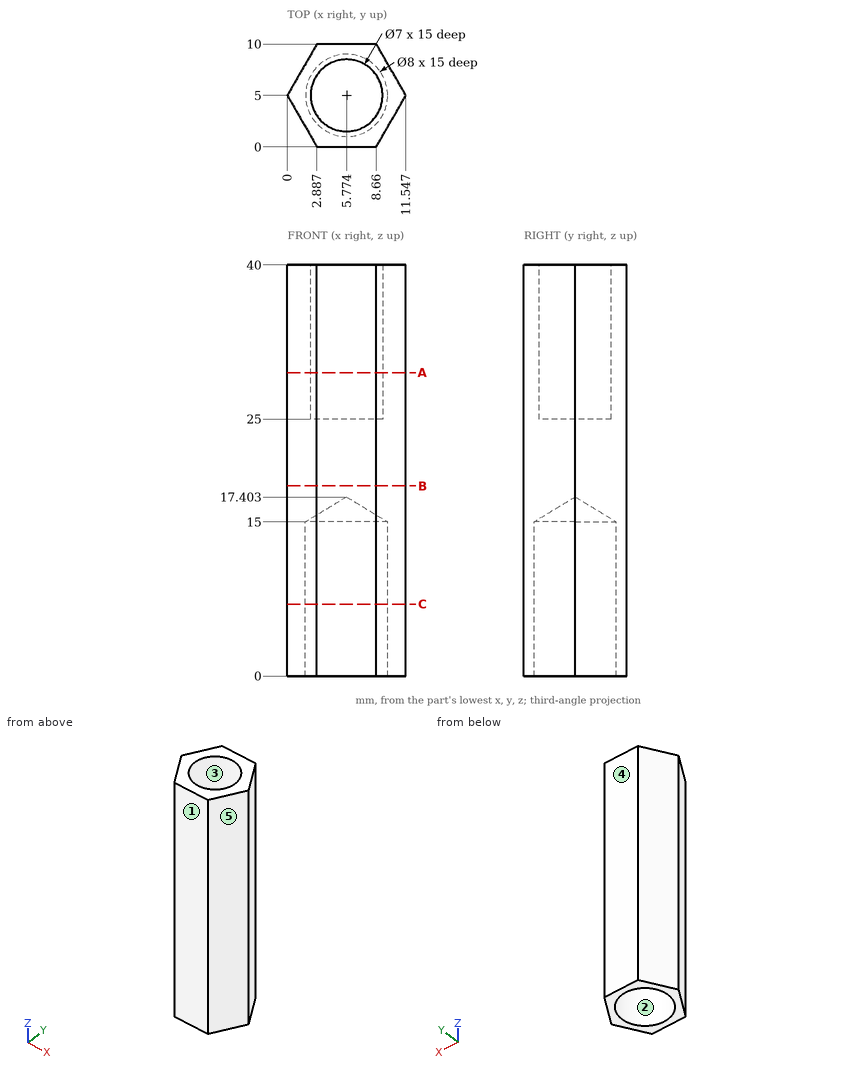
Here's the drawing with two shaded views (mm, measured from the low corner). I have some questions. A direction names the side the tool comes from. Coordinates: 2 decimals unless noted, no trailing zeros. Write each loop counter-clockwise with the first axis right and the second up, starting at its lowest first coordinate (ties: lowest second). Pieces come first, ordered by that corner, then holes. Notation, with made-up numbers: M -27,-25 L 17,-25 A29 cw 17,7 Z; hole C -9.5,4 d2. An arc over 180 degrees is marked long. Answer as CSV lines item,"result".
Item 1: Imagine slicing it at C-C on z = 7. List the corners of the cut face in (x, y) for me.
Geometry results:
outline,"M 0,5 L 2.89,0 L 8.66,0 L 11.55,5 L 8.66,10 L 2.89,10 Z; hole C 5.77,5 d8"
Item 2: I'm going to push flat-ended pins straight in: P1, Ø3.5, axis at x = 5.5, y = 5.5, coming from the +Z side; P2, Ø4, axis at y = 2.5, z = 8.5, coming from the +X side; P3, Ø5.5, axis at x = 5.77, y = 5, coming from the -Z side. Where does each tip first touch, or does it pass through?
Geometry results:
P1,"stops at z = 25"
P2,"stops at x = 11.26"
P3,"stops at z = 15.75"
Item 3: Imagine slicing it at B-B on z = 18.5. List the corners of the cut face in (x, y) for me, plus the area to 3 significant figures.
Geometry results:
outline,"M 0,5 L 2.89,0 L 8.66,0 L 11.55,5 L 8.66,10 L 2.89,10 Z"
area,"86.6 mm2"
Item 4: Please list where these lines run through material, in increasing order: line 1 along X through (y, z) = (5, 11) (1 decimal); line 2 along Y through (x, z) = (5.75, 2); line 3 along X through (y, z) = (3, 10) (1 decimal).
Geometry results:
line 1,"x = 0 to 1.8, 9.8 to 11.5"
line 2,"y = 0 to 1, 9 to 10"
line 3,"x = 1.2 to 2.3, 9.2 to 10.4"
Item 5: On a 3-axis mill with a long thin cutter (end or side, diameter ignored), from which of +Z, -Z, +X, -X, +Y, -Y can I reach the whole of each face in a straight line? I mean the marked faces 1 and 2. Say none if no direction works.
Geometry results:
face 1,"+Z, -Z, +X, -X, -Y"
face 2,"-Z"
Item 6: Imagine slicing it at A-A on z = 29.5. List the corners of the cut face in (x, y) for me.
Geometry results:
outline,"M 0,5 L 2.89,0 L 8.66,0 L 11.55,5 L 8.66,10 L 2.89,10 Z; hole C 5.77,5 d7"
Item 7: We'd pull the mould along Y, two halves only. Please class the marked faces 3, 4 and 5: +Y half, -Y half, draft (parallel to the pull), parting line (faces both ways), or undercut.
Geometry results:
face 3,"undercut"
face 4,"+Y half"
face 5,"-Y half"
